Source: CAD feature listing. Evaluate the final solid. Frame: model axes, mm. Face numbers are marked on the shaded views. A direction names the side the tool comes from. Round coordinates to 2 decimals unless told otherwise and drop trailing zeros. Order: outer loops, then holes, each group sorted by start corner. A loop starts at its lowest first (then second) coordinate and runs counter-clockwise, first axis right, second up. Notation, with made-up numbers: (63, 51.5) -> (74, 51.5) arc R25 cw to (74, 79.5) -> close; hole circle Ø2 at (-36.5, 44). An arc over 180 degrees is marked (long way). Answer as CSV lines item,"result". Start each with the question number.
(1) Section query A-A (x = 4.25). Output: boundary loops of the cut face in (y, z), plus the area to 3 significant figures.
(2) Set-up query: the marked faces 4, 5 and 6. Return all of +Z, -Z, +X, -X, +Y, -Y with unobstructed straight access to the full face (end or side cutting, diameter ignored); none if empty.
(3) Contact query for flat-ended pins moving along their axis: P1, Ø2, axis at x = 0, y = -1.5, coming from the +Z side; P2, Ø3, axis at x = 6.5, z = -2, coming from the +Y side; P3, Ø3, axis at x = 2.5, z = -2.5, coming from the -Y side. Output: stop coordinate, or through.
(4) Pull-direction query (Y, two-part tool) for the marked faces 1, 2 and 3; classes: +Y half, -Y half, draft (parallel to the pull), parting line (faces both ways), or undercut.
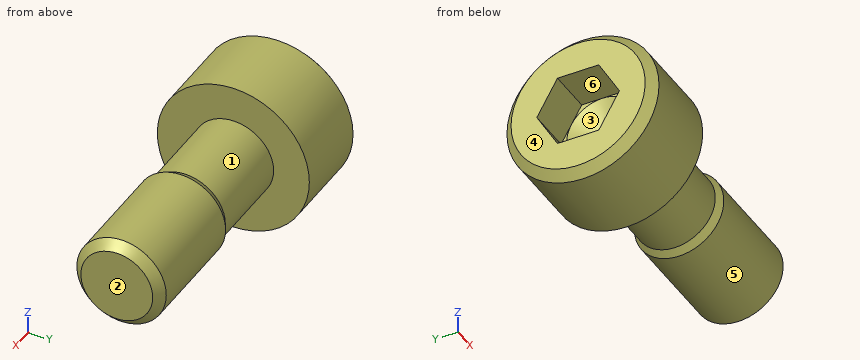
Autodesk Inventor part; units mm, degrees
ref_plane "bolt_to_spring_washer_XY" through (1.8, 0, 0) normal (1, 0, 0) x (0, 0, -1)
ref_plane "bolt_to_spring_washer_YZ" through (1.8, 0, 0) normal (0, 0, -1) x (0, 1, 0)
ref_plane "bolt_to_spring_washer_ZX" through (1.8, 0, 0) normal (0, 1, 0) x (1, 0, 0)
sketch "Sketch_6" plane through (0, 0, 0) normal (0, 0, 1) x (1, 0, 0)
  line L0 (12, 0) -> (4.5504, 0)
  line L1 (4.5504, 0) -> (4.5504, 2.0095)
  line L2 (4.5504, 2.0095) -> (5.4, 2.5)
  line L3 (5.4, 2.5) -> (11.5095, 2.5)
  line L4 (11.5095, 2.5) -> (12, 2.0095)
  line L5 (12, 2.0095) -> (12, 0)
  line L6 (12, 0) -> (4.5504, 0)
revolve "Revolution1" add sketch "Sketch_6" angle 360 about axis through (12, 0, 0) along (1, 0, 0)
thread "Thread1"
sketch "Sketch_1" plane through (0, 0, 0) normal (0, 0, 1) x (1, 0, 0)
  line L0 (5.4, 0) -> (-5, 0)
  line L1 (-1.3453, 0) -> (-2.5, 2)
  line L2 (-2.5, 2) -> (-5, 2)
  line L3 (-5, 2) -> (-5, 3.75)
  line L4 (-5, 3.75) -> (-4.5, 4.25)
  line L5 (-4.5, 4.25) -> (0, 4.25)
  line L6 (0, 4.25) -> (0, 2.2543)
  line L7 (0, 2.2543) -> (5.4, 2.2543)
  line L8 (5.4, 2.2543) -> (5.4, 0)
  line L9 (5.4, 0) -> (-1.3453, 0)
revolve "Revolution2" add sketch "Sketch_1" angle 360 about axis through (5.4, 0, 0) along (1, 0, 0)
sketch "Sketch_2" plane through (-5, 0, 0) normal (1, 0, 0) x (0, 0, -1)
  line L0 (-2, 1.1547) -> (-2, -1.1547)
  line L1 (-2, -1.1547) -> (0, -2.3094)
  line L2 (0, -2.3094) -> (2, -1.1547)
  line L3 (2, -1.1547) -> (2, 1.1547)
  line L4 (2, 1.1547) -> (0, 2.3094)
  line L5 (0, 2.3094) -> (-2, 1.1547)
extrude "Extrusion1" cut sketch "Sketch_2" along normal blind 2.5
ref_plane "bolt_to_spring_washer_XY" through (1.8, 0, 0) normal (1, 0, 0) x (0, 0, -1)
ref_plane "bolt_to_spring_washer_YZ" through (1.8, 0, 0) normal (0, 0, -1) x (0, 1, 0)
ref_plane "bolt_to_spring_washer_ZX" through (1.8, 0, 0) normal (0, 1, 0) x (1, 0, 0)
ref_plane "bolt_to_plane_washer_XY" through (3.6, 0, 0) normal (1, 0, 0) x (0, 0, -1)
ref_plane "bolt_to_plane_washer_YZ" through (3.6, 0, 0) normal (0, 0, -1) x (0, 1, 0)
ref_plane "bolt_to_plane_washer_ZX" through (3.6, 0, 0) normal (0, 1, 0) x (1, 0, 0)
ref_plane "screw_to_body_XY" through (0, 0, 0) normal (1, 0, 0) x (0, 0, -1)
ref_plane "screw_to_body_YZ" through (0, 0, 0) normal (0, 0, -1) x (0, 1, 0)
ref_plane "screw_to_body_ZX" through (0, 0, 0) normal (0, 1, 0) x (1, 0, 0)
properties part number "HCBST5-12_Screw"
Answer block:
1,outline,"circle Ø4.51 at (0, 0)"
1,area,"16.0 mm2"
2,face 4,"+Z, -Z, -X, +Y, -Y"
2,face 5,"+X"
2,face 6,"-X"
3,P1,"z = 4.22"
3,P2,"y = 2.45"
3,P3,"y = -2.02"
4,face 1,"parting line"
4,face 2,"draft"
4,face 3,"undercut"
